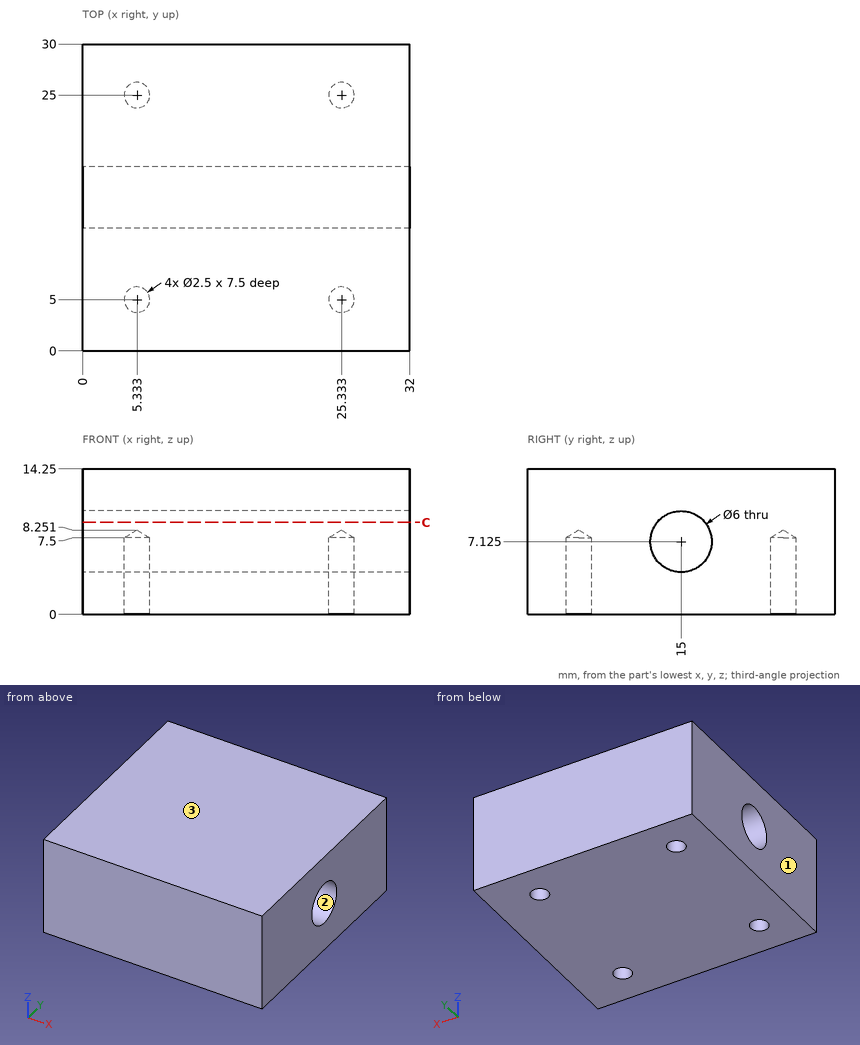
Verification items for this drawing (mm, ordinates from the low corner). Give positions to 0.01 mm unless a question says otherwise; leave off trailing zeros. Write each loop counter-clockwise with the first axis right and the second up, starting at its lowest first coordinate (ties: lowest second). Pieces come first, ordered by that corner, then holes. Notation, with made-up numbers: (5.5, -23.75) - (39.5, -23.75) arc R20 cw to (39.5, -2.75) - close; hole circle Ø5 at (82, 12.25). An arc over 180 degrees is marked (long way). Answer as a JSON object with one key per item and string values. Group by question number.
1) Release check for a two-part mould opening along Z. For the marked faces 1, 2 and 3 record: pulls with the +Z half, pulls with the -Z half, needs draft (parallel to the pull), parting line crosses it, or undercut.
2) Sectioned sample at C-C (z = 9). Record the cut outline in (x, y).
3) Thickness scan on probe 1 along X at (y, z) = (5, 5); probe 2 along Y at (x, z) = (5, 4.75) (1 decimal); probe 3 along Z at (x, y) = (20, 16.25). Record the ranges inside material, lowest first. Write a range as from..to.
Geometry results:
{
 "1": {"face 1": "needs draft", "face 2": "undercut", "face 3": "pulls with the +Z half"},
 "2": {"outline": "(0, 0) - (32, 0) - (32, 12.66) - (0, 12.66) - close; (0, 17.34) - (32, 17.34) - (32, 30) - (0, 30) - close"},
 "3": {"probe 1": "x = 0..4.08, 6.58..24.08, 26.58..32", "probe 2": "y = 0..3.8, 6.2..13.2, 16.8..23.8, 26.2..30", "probe 3": "z = 0..4.4, 9.85..14.25"}
}
